from build123d import *

# Parameters (mm, degrees)
ESQUISSE1_W             = 432.465319529
ESQUISSE1_H             = 1000
BOSS_EXTRU_1_DEPTH      = 15
ESQUISSE2_W             = 15
ESQUISSE2_H             = 180
ENL_V_MAT_EXTRU_1_DEPTH = 1090.610596771
ESQUISSE3_W             = 15
ESQUISSE3_H             = 386.42955672
ENL_V_MAT_EXTRU_2_DEPTH = 928.173798484
ESQUISSE4_W             = 42
ESQUISSE4_H             = 42.455270474
ENL_V_MAT_EXTRU_3_DEPTH = 863.948765929
ENL_V_MAT_EXTRU_4_DEPTH = 7
ESQUISSE6_R             = 7.5
ENL_V_MAT_EXTRU_5_DEPTH = 863.85547609


with BuildPart() as part:
    # Esquisse1 → Boss.-Extru.1 (new body)
    with BuildSketch(Plane.XY):
        with Locations((-52.199031023, -500)):
            Rectangle(ESQUISSE1_W, ESQUISSE1_H)
    extrude(amount=BOSS_EXTRU_1_DEPTH)

    # Esquisse2 → Enlèv. mat.-Extru.1 (cut, through all)
    with BuildSketch(Plane(origin=(164.033628742, 0, 0), x_dir=(0, 0, -1), z_dir=(1, 0, 0))):
        with Locations((-7.5, -910)):
            Rectangle(ESQUISSE2_W, ESQUISSE2_H)
    extrude(amount=-ENL_V_MAT_EXTRU_1_DEPTH, mode=Mode.SUBTRACT)

    # Esquisse3 → Enlèv. mat.-Extru.2 (cut, through all)
    with BuildSketch(Plane.ZY.offset(268.431690787)):
        with Locations((7.5, -193.21477836)):
            Rectangle(ESQUISSE3_W, ESQUISSE3_H)
    extrude(amount=-ENL_V_MAT_EXTRU_2_DEPTH, mode=Mode.SUBTRACT)

    # Esquisse4 → Enlèv. mat.-Extru.3 (cut, through all)
    with BuildSketch(Plane(origin=(0, 0, 0), x_dir=(-1, 0, 0), z_dir=(0, 0, -1))):
        with Locations((52.199031023, -799)):
            Rectangle(ESQUISSE4_W, ESQUISSE4_H)
    extrude(amount=-ENL_V_MAT_EXTRU_3_DEPTH, mode=Mode.SUBTRACT)

    # Esquisse5 → Enlèv. mat.-Extru.4 (cut)
    with BuildSketch(Plane(origin=(0, 0, 0), x_dir=(-1, 0, 0), z_dir=(0, 0, -1))):
        with BuildLine():
            ThreePointArc((52.199031023, -418.42955672), (63.199031023, -407.42955672), (52.199031023, -396.42955672))
            ThreePointArc((52.199031023, -396.42955672), (41.199031023, -407.42955672), (52.199031023, -418.42955672))
        make_face()
    extrude(amount=-ENL_V_MAT_EXTRU_4_DEPTH, mode=Mode.SUBTRACT)

    # Esquisse6 → Enlèv. mat.-Extru.5 (cut, through all)
    with BuildSketch(Plane(origin=(0, 0, 7), x_dir=(-1, 0, 0), z_dir=(0, 0, -1))):
        with Locations((52.199031023, -407.42955672)):
            Circle(ESQUISSE6_R)
    extrude(amount=-ENL_V_MAT_EXTRU_5_DEPTH, mode=Mode.SUBTRACT)


solid = part.part
Work out the finished part from the listing and answer in its coordinate system (mm). A direction names the side the tool comes from. Coordinates: 2 decimals unless noted, no trailing zeros.
1. Consider line 1 along X through (y, z) = (-796, 5); line 2 along Y through (x, z) = (-37, 13); line 3 along Y through (x, z) = (-44, 1.5). Determine where each line is inside the solid, lowest interval first.
Results list:
line 1: x = -268.43 to -73.2, -31.2 to 164.03
line 2: y = -777.77 to -386.43
line 3: y = -777.77 to -414.76, -400.1 to -386.43
2. For faces 4 (the flat face through (-169, -820, 8)), 5 (the flat face through (-54, -415, 7)), 6 (the flat face through (-52, -777.772, 7)), determine the directions among +Z, -Z, +X, -X, +Y, -Y from which every point of the face is accessible in a straight line to the end or side of a thin tool.
Results list:
face 4: +Z, -Z, +X, -X, -Y
face 5: -Z
face 6: +Z, -Z, -Y
3. Flat-ended cylindrical pins translate along their axes: pin 1 (11 mm diameter, centred on x = -53.5, y = -409, fed in from -Z); pin 2 (7.5 mm diameter, centred on x = -48.5, z = 5, fed in from -Y); pin 3 (13.5 mm diameter, centred on x = -52.2, y = -407.43, fed in from +Z). Find the tip coordinate at first contact, or state that the pin passes through.
Results list:
pin 1: stops at z = 7
pin 2: stops at y = -777.77
pin 3: passes through
4. For a pull along Y with two mould halves and no side action, classify faces 1 (the flat face through (164.034, -606, 7)), 2 (the flat face through (-55, -386.43, 7)), 3 (the cylindrical face through (-56.412, -397.268, 3.451)) as +Y half, -Y half, draft (parallel to the pull), parting line (faces both ways), or undercut.
Results list:
face 1: draft
face 2: +Y half
face 3: undercut
